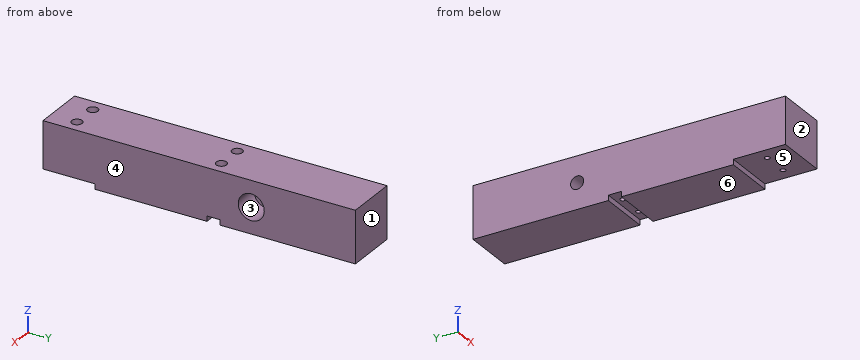
```python
from build123d import *

# Parameters (mm, degrees)
SKETCH1_W           = 20
SKETCH1_H           = 120
SKETCH1_R           = 2.5
BOSS_EXTRUDE2_DEPTH = 20
SKETCH10_R          = 5
CUT_EXTRUDE1_DEPTH  = 10
SKETCH11_R          = 1
CUT_EXTRUDE2_DEPTH  = 21
SKETCH12_R          = 2
CUT_EXTRUDE3_DEPTH  = 5
SKETCH11_3_R        = 1
CUT_EXTRUDE4_DEPTH  = 21
SKETCH14_W          = 20
SKETCH14_H          = 5
SKETCH14_H_2        = 20
CUT_EXTRUDE6_DEPTH  = 2


with BuildPart() as part:
    # Sketch1 → Boss-Extrude2 (new body)
    with BuildSketch(Plane(origin=(0, 0, 0), x_dir=(0, 0, -1), z_dir=(1, 0, 0))):
        with Locations((10, 60)):
            Rectangle(SKETCH1_W, SKETCH1_H)
        with Locations((10, 80)):
            Circle(SKETCH1_R, mode=Mode.SUBTRACT)
    extrude(amount=-BOSS_EXTRUDE2_DEPTH)

    # Sketch10 → Cut-Extrude1 (cut)
    with BuildSketch(Plane(origin=(0, 0, 0), x_dir=(0, 0, -1), z_dir=(1, 0, 0))):
        with Locations((10, 80)):
            Circle(SKETCH10_R)
    extrude(amount=-CUT_EXTRUDE1_DEPTH, mode=Mode.SUBTRACT)

    # Sketch11 → Cut-Extrude2 (cut, through all)
    with BuildSketch(Plane.XY):
        with Locations((-15, 10)):
            Circle(SKETCH11_R)
        with Locations((-5, 10)):
            Circle(SKETCH11_R)
    extrude(amount=-CUT_EXTRUDE2_DEPTH, mode=Mode.SUBTRACT)

    # Sketch12 → Cut-Extrude3 (cut)
    with BuildSketch(Plane.XY):
        with Locations((-15, 10)):
            Circle(SKETCH12_R)
        with Locations((-5, 10)):
            Circle(SKETCH12_R)
        with Locations((-15, 65.5)):
            Circle(SKETCH12_R)
        with Locations((-5, 65.5)):
            Circle(SKETCH12_R)
    extrude(amount=-CUT_EXTRUDE3_DEPTH, mode=Mode.SUBTRACT)

    # Sketch11<3> → Cut-Extrude4 (cut, through all)
    with BuildSketch(Plane.XY):
        with Locations((-15, 65.5)):
            Circle(SKETCH11_3_R)
        with Locations((-5, 65.5)):
            Circle(SKETCH11_3_R)
    extrude(amount=-CUT_EXTRUDE4_DEPTH, mode=Mode.SUBTRACT)

    # Sketch14 → Cut-Extrude6 (cut)
    with BuildSketch(Plane(origin=(0, 0, -20), x_dir=(-1, 0, 0), z_dir=(0, 0, -1))):
        with Locations((10, 65.5)):
            Rectangle(SKETCH14_W, SKETCH14_H)
        with Locations((10, 10)):
            Rectangle(SKETCH14_W, SKETCH14_H_2)
    extrude(amount=-CUT_EXTRUDE6_DEPTH, mode=Mode.SUBTRACT)


solid = part.part
```
Read the model definition and answer for the solid it produces. Units are mm, in the model's axes. Face numbers are marked on the shaded views. A direction names the side the tool comes from. Coordinates: 2 decimals unless noted, no trailing zeros. Loops run counter-clockwise (first coordinate to the right, second up) from the corner with the lowest first, then second, coordinate; pieces in that order, holes last. Notation, with made-up numbers: (36, 48.25) -> (49, 48.25) arc R22 ccw to (49, 62.25) -> close; hole circle Ø8 at (18, 23.5). An arc over 180 degrees is marked (long way). Return JSON: item names as keys, results as strings.
Item 1: For a pull along Y with two mould halves and no side action, classify the marked faces 1, 2, 3 and 4 as +Y half, -Y half, draft (parallel to the pull), parting line (faces both ways), or undercut.
Answers:
{"face 1": "+Y half", "face 2": "-Y half", "face 3": "undercut", "face 4": "draft"}
Item 2: For the marked faces 5 and 6, determine the directions among +Z, -Z, +X, -X, +Y, -Y from which every point of the face is accessible in a straight line to the end or side of a thin tool.
Answers:
{"face 5": "-Z, +X, -X, -Y", "face 6": "-Z, +X, -X, +Y, -Y"}
Item 3: Find section A-A (x = -15). Determine the outline of the cut face in (y, z), plus the area to 3 significant figures.
Answers:
{"outline": "(0, -18) -> (9, -18) -> (9, -5) -> (8, -5) -> (8, 0) -> (0, 0) -> close; (11, -18) -> (20, -18) -> (20, -20) -> (63, -20) -> (63, -18) -> (64.5, -18) -> (64.5, -5) -> (63.5, -5) -> (63.5, 0) -> (12, 0) -> (12, -5) -> (11, -5) -> close; (66.5, -18) -> (68, -18) -> (68, -20) -> (120, -20) -> (120, 0) -> (67.5, 0) -> (67.5, -5) -> (66.5, -5) -> close; hole circle Ø5 at (80, -10)", "area": "2,240 mm2"}
Item 4: Find the intervals of material crossed by probe 1 along X at (y, z) = (65.5, -15.25); probe 2 along Y at (x, z) = (-5, -12.25); probe 3 along Y at (x, z) = (-15, -9), in increasing order.
Answers:
{"probe 1": "x = -20 to -16, -14 to -6, -4 to 0", "probe 2": "y = 0 to 9, 11 to 64.5, 66.5 to 75.53, 84.47 to 120", "probe 3": "y = 0 to 9, 11 to 64.5, 66.5 to 77.71, 82.29 to 120"}
Item 5: Find section B-B (z = -9). Determine the outline of the cut face in (x, y).
Answers:
{"outline": "(-20, 0) -> (0, 0) -> (0, 75.1) -> (-10, 75.1) -> (-10, 77.71) -> (-20, 77.71) -> close; (-20, 82.29) -> (-10, 82.29) -> (-10, 84.9) -> (0, 84.9) -> (0, 120) -> (-20, 120) -> close; hole circle Ø2 at (-15, 10); hole circle Ø2 at (-15, 65.5); hole circle Ø2 at (-5, 10); hole circle Ø2 at (-5, 65.5)"}
Item 6: Flat-ended cylindrical pins translate along their axes: P1, Ø3, axis at x = -15, y = 65.5, coming from the -Z side; P2, Ø1.2, axis at x = -14, y = 9.5, coming from the +Z side; P3, Ø0.6, axis at x = -7, z = -19.5, coming from the -Y side; P4, Ø4, axis at y = 80, z = -10, coming from the -X side. Find the tip coordinate at first contact, or state that the pin passes through.
Answers:
{"P1": "stops at z = -18", "P2": "stops at z = -5", "P3": "stops at y = 20", "P4": "passes through"}
Item 7: Find section D-D (x = -2). Determine the outline of the cut face in (y, z), plus the area to 3 significant figures.
Answers:
{"outline": "(0, -18) -> (20, -18) -> (20, -20) -> (63, -20) -> (63, -18) -> (68, -18) -> (68, -20) -> (120, -20) -> (120, 0) -> (0, 0) -> close; hole circle Ø10 at (80, -10)", "area": "2,270 mm2"}
Item 8: Find section C-C (y = 10). Determine the outline of the cut face in (x, z), plus the area to 3 significant figures.
Answers:
{"outline": "(-20, -18) -> (-16, -18) -> (-16, -5) -> (-17, -5) -> (-17, 0) -> (-20, 0) -> close; (-14, -18) -> (-6, -18) -> (-6, -5) -> (-7, -5) -> (-7, 0) -> (-13, 0) -> (-13, -5) -> (-14, -5) -> close; (-4, -18) -> (0, -18) -> (0, 0) -> (-3, 0) -> (-3, -5) -> (-4, -5) -> close", "area": "268 mm2"}
